CAD build for the part. Positions are in the model's coordinates, mm. A direction names the side the tool comes from. Give positions to 0.01 mm unless a question says otherwise; leave off trailing zeros. Answer as a JSON object with one key per item and string values.
from build123d import *

# Parameters (mm, degrees)
SKETCH1_W           = 130
SKETCH1_H           = 82
BOSS_EXTRUDE1_DEPTH = 5
SKETCH3_W           = 130
SKETCH3_H           = 82
SKETCH2_W           = 120
SKETCH2_H           = 46
CHAMFER1_SIZE       = 2
SKETCH4_R           = 1.2
CUT_EXTRUDE1_DEPTH  = 6
SKETCH5_W           = 114
SKETCH5_H           = 40
CUT_EXTRUDE2_DEPTH  = 21
SKETCH6_W           = 118
SKETCH6_H           = 56
CUT_EXTRUDE3_DEPTH  = 12
SKETCH8_W           = 7
SKETCH8_H           = 7
BOSS_EXTRUDE2_DEPTH = 8
SKETCH9_R           = 2.1
CUT_EXTRUDE4_DEPTH  = 8
SKETCH10_W          = 2
SKETCH10_H          = 40
CUT_EXTRUDE5_DEPTH  = 9
FILLET1_R           = 3


with BuildPart() as part:
    # Sketch1 → Boss-Extrude1 (new body)
    with BuildSketch(Plane(origin=(0, 0, 0), x_dir=(1, 0, 0), z_dir=(0, 1, 0))):
        Rectangle(SKETCH1_W, SKETCH1_H)
    extrude(amount=BOSS_EXTRUDE1_DEPTH)

    # Sketch3 → Loft2 section 0
    with BuildSketch(Plane(origin=(0, 5, 0), x_dir=(1, 0, 0), z_dir=(0, 1, 0))):
        Rectangle(SKETCH3_W, SKETCH3_H)
    # Sketch2 → Loft2 section 1
    with BuildSketch(Plane(origin=(0, 22, 0), x_dir=(1, 0, 0), z_dir=(0, 1, 0))):
        Rectangle(SKETCH2_W, SKETCH2_H)
    loft()

    # Chamfer1
    chamfer1_edges = [part.edges().sort_by_distance(p)[0] for p in [
        (-65, 2.5, 41),
        (65, 2.5, 41),
        (65, 2.5, -41),
        (-65, 2.5, -41),
    ]]
    chamfer(chamfer1_edges, length=CHAMFER1_SIZE)

    # Sketch4 → Cut-Extrude1 (cut)
    with BuildSketch(Plane.XZ):
        with Locations((40, -37.5)):
            Circle(SKETCH4_R)
        with Locations((-40, -37.5)):
            Circle(SKETCH4_R)
    cut_extrude1 = extrude(amount=-CUT_EXTRUDE1_DEPTH, mode=Mode.SUBTRACT)

    # Sketch5 → Cut-Extrude2 (cut)
    with BuildSketch(Plane.XZ):
        Rectangle(SKETCH5_W, SKETCH5_H)
    extrude(amount=-CUT_EXTRUDE2_DEPTH, mode=Mode.SUBTRACT)

    # Mirror1: Cut-Extrude1 across plane
    add(cut_extrude1.mirror(Plane.XY), mode=Mode.SUBTRACT)

    # Sketch6 → Cut-Extrude3 (cut)
    with BuildSketch(Plane.XZ):
        Rectangle(SKETCH6_W, SKETCH6_H)
    extrude(amount=-CUT_EXTRUDE3_DEPTH, mode=Mode.SUBTRACT)

    # Sketch8 → Boss-Extrude2 (add)
    with BuildSketch(Plane(origin=(0, 4, 0), x_dir=(-1, 0, 0), z_dir=(0, -1, 0))):
        with Locations((-55.5, 24.5)):
            Rectangle(SKETCH8_W, SKETCH8_H)
        with Locations((-55.5, -24.5)):
            Rectangle(SKETCH8_W, SKETCH8_H)
        with Locations((55.5, -24.5)):
            Rectangle(SKETCH8_W, SKETCH8_H)
        with Locations((55.5, 24.5)):
            Rectangle(SKETCH8_W, SKETCH8_H)
    extrude(amount=-BOSS_EXTRUDE2_DEPTH)

    # Sketch9 → Cut-Extrude4 (cut)
    with BuildSketch(Plane.XZ.offset(-4)):
        with Locations((-55.5, 24.5)):
            Circle(SKETCH9_R)
        with Locations((55.5, 24.5)):
            Circle(SKETCH9_R)
        with Locations((55.5, -24.5)):
            Circle(SKETCH9_R)
        with Locations((-55.5, -24.5)):
            Circle(SKETCH9_R)
    extrude(amount=-CUT_EXTRUDE4_DEPTH, mode=Mode.SUBTRACT)

    # Sketch10 → Cut-Extrude5 (cut)
    with BuildSketch(Plane.XZ.offset(-12)):
        with Locations((-58, 0)):
            Rectangle(SKETCH10_W, SKETCH10_H)
        with Locations((58, 0)):
            Rectangle(SKETCH10_W, SKETCH10_H)
    extrude(amount=-CUT_EXTRUDE5_DEPTH, mode=Mode.SUBTRACT)

    # Fillet1
    fillet1_edges = [part.edges().sort_by_distance(p)[0] for p in [
        (0, 5, 41),
        (0, 5, -41),
    ]]
    fillet(fillet1_edges, radius=FILLET1_R)


solid = part.part
(1) Pull direction Z, two halves, no side cores. Call faces 3 (the face through (0, 0, -31)), 4 (the face through (-1, 2, 41)), 5 (the face through (40.65, 2.96, 36.49)): pulls with the +Z half, pulls with the -Z half, needs draft (parallel to the pull), parting line crosses it, or undercut.
Answer key:
{"face 3": "needs draft", "face 4": "pulls with the +Z half", "face 5": "undercut"}
(2) Probe L1, parallel to X at y = 2.6, z = 37.5; L2, parallel to X at y = 1.25, z = 15; L3, parallel to Y at x = -39, z = 17.5. List the from-to ranges inside material, lowest first. Write a range as [from, to].
Answer key:
{"L1": "x = [-65, -41.2], [-38.8, 38.8], [41.2, 65]", "L2": "x = [-65, -59], [59, 65]", "L3": "y = [21, 22]"}
(3) 3-axis set-ups, long thin cutter, end or side, ignore diameter. For faces 1 (the face through (57.1, 4, 22.9)), 2 (the face through (-1, 2, -41)): which of +Z, -Z, +X, -X, +Y, -Y reach the whole face in a straight line?
Answer key:
{"face 1": "-Y", "face 2": "-Z, +X, -X, +Y, -Y"}
(4) Flat gauge pins, fed straight in: P1, Ø3.5, axis at x = -55.5, y = 7.5, coming from the +Z side; P2, Ø2, axis at x = -40, z = -37.5, coming from the -Y side; P3, Ø6, axis at x = 18.5, z = 29.5, coming from the +Y side. Where does each tip first touch, or does it go through?
Answer key:
{"P1": "stops at z = 40.2", "P2": "stops at y = 6", "P3": "stops at y = 18.69"}
